```python
from build123d import *

# Parameters (mm, degrees)
SKETCH2_R          = 23.5
SKETCH2_R_2        = 16
SKETCH3_R          = 3.1
CUT_EXTRUDE1_DEPTH = 40


with BuildPart() as part:
    # Sweep8: sweep along a path in Sketch1
    with BuildLine(Plane(origin=(0, 0, 0), x_dir=(1, 0, 0), z_dir=(0, 1, 0))) as sweep8_path:
        Line((0, 0), (0, 30))
        ThreePointArc((0, 30), (8.786796564, 51.213203436), (30, 60))
        Line((30, 60), (60, 60))
    # Sketch2 → Sweep8 (sweep)
    with BuildSketch(Plane.XY):
        Circle(SKETCH2_R)
        Circle(SKETCH2_R_2, mode=Mode.SUBTRACT)
    sweep(path=sweep8_path.line)

    # Sketch3 → Cut-Extrude1 (cut)
    with BuildSketch(Plane(origin=(0, 0, 0), x_dir=(1, 0, 0), z_dir=(0, 1, 0))):
        with Locations((0, 15)):
            Circle(SKETCH3_R)
        with Locations((45, 60)):
            Circle(SKETCH3_R)
    extrude(amount=CUT_EXTRUDE1_DEPTH, mode=Mode.SUBTRACT)


solid = part.part
```
Source: CAD feature listing. Evaluate the final solid. Frame: model axes, mm. A direction names the side the tool comes from. Coordinates: 2 decimals unless noted, no trailing zeros. Loops run counter-clockwise (first coordinate to the right, second up) from the corner with the lowest first, then second, coordinate; pieces in that order, holes last. Notation, with made-up numbers: (58, 55) - (95, 55) arc R20 ccw to (95, 73) - close; hole circle Ø1 at (32.25, 61.25). An arc over 180 degrees is marked (long way). Answer as CSV lines item,"result".
1. Section B-B (x = 34). Return loops of the section in (y, z), then the cut area to 3 significant figures.
Established:
outline,"circle Ø47 at (0, -60); hole circle Ø32 at (0, -60)"
area,"931 mm2"
2. Contact query for flat-ended pins moving along their axis: pin 1 (2 mm diameter, centred on y = 14.5, z = -54.5, fed in from +X); pin 2 (8 mm diameter, centred on y = -11, z = -33.5, fed in from +X); pin 3 (6 mm diameter, centred on x = 38, y = -14, fed in from -Z); pin 4 (3 mm diameter, centred on y = 16, z = -17, fed in from -X). Output: stop coordinate, or through.
Established:
pin 1,"stops at x = 60"
pin 2,"stops at x = 25.51"
pin 3,"stops at z = -80.77"
pin 4,"stops at x = -18.49"
3. Ray query, line 1 (Y direction, x = 51, z = -60); line 2 (Z direction, x = 52.5, y = 0.5); line 3 (X direction, y = -4, z = -30.5). Return the intervals inside material, ascending.
Established:
line 1,"y = -23.5 to -16, 16 to 23.5"
line 2,"z = -83.49 to -75.99, -44.01 to -36.51"
line 3,"x = -23.15 to -15.49, 15.5 to 23.18"
4. Section A-A (y = 0). Return loops of the section in (x, z).
Established:
outline,"(-23.5, -30) arc R53.5 ccw to (30, -83.5) - (60, -83.5) - (60, -76) - (30, -76) arc R46 cw to (-16, -30) - (-16, 0) - (-23.5, 0) - close; (16, -30) arc R14 ccw to (30, -44) - (60, -44) - (60, -36.5) - (30, -36.5) arc R6.5 cw to (23.5, -30) - (23.5, 0) - (16, 0) - close"
5. Section C-C (z = -10.5). Return loops of the section in (x, y).
Established:
outline,"circle Ø47 at (0, 0); hole circle Ø32 at (0, 0)"
6. Reachability of faces 4 (the flat face through (-6, -15, 0)), 5 (the cylindrical face through (-3.47, 15.62, -15.21)), 6 (the cylindrical face through (46.67, 19.54, -62.61)) from +Z, -Z, +X, -X, +Y, -Y: full face, straight path, thin tool, end or side. Return the list, or none.
Established:
face 4,"+Z, +X, -X, +Y, -Y"
face 5,"+Z"
face 6,"+Y"
7. Section D-D (y = 9.5). Return loops of the section in (x, z).
Established:
outline,"(-21.49, -30) arc R51.49 ccw to (30, -81.49) - (60, -81.49) - (60, -72.87) - (30, -72.87) arc R42.87 cw to (-12.87, -30) - (-12.87, 0) - (-21.49, 0) - close; (12.87, -30) arc R17.13 ccw to (30, -47.13) - (60, -47.13) - (60, -38.51) - (30, -38.51) arc R8.51 cw to (21.49, -30) - (21.49, 0) - (12.87, 0) - close"
8. Mould query, pull axis Y, two halves, no side actions, for faces 1 (the cylindrical face through (45.21, -0.703, -75.985)), 2 (the cylindrical face through (45.21, -1.033, -83.477)), 3 (the flat face through (60, -6, -75)). Classes: released by +Y, released by -Y, zero draft, split by the parting line, or undercut.
Established:
face 1,"undercut"
face 2,"split by the parting line"
face 3,"zero draft"
